CAD build for the part. Positions are in the model's coordinates, mm. A direction names the side the tool comes from. Coordinates: 2 decimals unless noted, no trailing zeros. Order: outer loops, then holes, each group sorted by start corner. A loop starts at its lowest first (then second) coordinate and runs counter-clockwise, first axis right, second up. Notation, with made-up numbers: (69, 68) - (81, 68) arc R30 ccw to (81, 102) - close; hole circle Ø4 at (23, 30.25). An arc over 180 degrees is marked (long way). Use one line per item in the form item = value.
```python
from build123d import *

# Parameters (mm, degrees)
SKETCH030_R             = 14.5
PAD018_DEPTH            = 47
SKETCH031_R             = 1.5875
PAD019_DEPTH            = 15
POCKET012_DEPTH         = 5
SKETCH033_R             = 5.5
PAD020_DEPTH            = 11
SKETCH034_R             = 33.5
PAD021_DEPTH            = 26
SKETCH035_R             = 1.5
POCKET013_DEPTH         = 7.5
SKETCH036_R             = 23
SKETCH036_R_2           = 5.5
POCKET014_DEPTH         = 11
BODY010_PLACEMENT_ANGLE = 180


with BuildPart() as part:
    # Sketch030 → Pad018 (new body)
    with BuildSketch(Plane.XZ):
        Circle(SKETCH030_R)
    extrude(amount=PAD018_DEPTH)

    # Sketch031 → Pad019 (join)
    with BuildSketch(Plane.XZ):
        Circle(SKETCH031_R)
    extrude(amount=-PAD019_DEPTH)

    # Sketch032 → Pocket012 (cut, symmetric)
    with BuildSketch(Plane.YZ):
        Polygon((3, 1.214123), (15, 1.214123), (15, 1.59), (2.863192, 1.59), align=None)
    extrude(amount=POCKET012_DEPTH, both=True, mode=Mode.SUBTRACT)

    # Sketch033 (on Face5 of Pocket012) → Pad020 (join)
    with BuildSketch(Plane(origin=(0, 15, 0), x_dir=(1, 0, 0), z_dir=(0, 1, 0))):
        Circle(SKETCH033_R)
    extrude(amount=-PAD020_DEPTH)

    # Sketch034 (on DatumPlane) → Pad021 (join)
    with BuildSketch(Plane.XZ.offset(-8)):
        Circle(SKETCH034_R)
    extrude(amount=-PAD021_DEPTH)

    # Sketch035 → Pocket013 (cut)
    with BuildSketch(Plane.XZ):
        with Locations((0, -9.5)):
            Circle(SKETCH035_R)
        with Locations((8, 0)):
            Circle(SKETCH035_R)
        with Locations((0, 9.5)):
            Circle(SKETCH035_R)
        with Locations((-8, 0)):
            Circle(SKETCH035_R)
    extrude(amount=POCKET013_DEPTH, mode=Mode.SUBTRACT)

    # Sketch036 (on DatumPlane) → Pocket014 (cut)
    with BuildSketch(Plane.XZ.offset(-8)):
        Circle(SKETCH036_R)
        Circle(SKETCH036_R_2, mode=Mode.SUBTRACT)
    extrude(amount=-POCKET014_DEPTH, mode=Mode.SUBTRACT)


with BuildPart() as part_1:
    # Body010 placement: moved
    add(part.part.moved(Location((-1, -113, 22.5))).rotate(Axis((-1, -113, 22.5), (0, 0, 1)), BODY010_PLACEMENT_ANGLE))


solid = part_1.part
```
Item 1: Cut at C-C, the plane z = 32. Write the cut outline in (x, y), plus the area to 3 significant figures.
Derived:
outline = (-33.12, -147) - (31.12, -147) - (31.12, -121) - (19.95, -121) - (19.95, -132) - (-21.95, -132) - (-21.95, -121) - (-33.12, -121) - close; (-11.95, -113) - (-2.5, -113) - (-2.5, -105.5) - (0.5, -105.5) - (0.5, -113) - (9.95, -113) - (9.95, -66) - (-11.95, -66) - close
area = 2,220 mm²
Item 2: Drop flat-ended pins along their axis: pin 1 (12 mm diameter, centred on x = -22.5, z = 7.5, fed in from +Y); pin 2 (12 mm diameter, centred on x = -13.5, y = -103, fed in from +Z); pin 3 (3 mm diameter, centred on y = -121.5, z = 9, fed in from +X). Give the stop position or say it passes through.
Derived:
pin_1 = -121
pin_2 = 35.46
pin_3 = 30.28
Item 3: Cut at D-D, the plane z = 22.5. Write the cut outline in (x, y).
Derived:
outline = (-34.5, -147) - (32.5, -147) - (32.5, -121) - (22, -121) - (22, -132) - (4.5, -132) - (4.5, -117) - (0.59, -117) - (0.59, -113) - (5.5, -113) - (5.5, -105.5) - (8.5, -105.5) - (8.5, -113) - (13.5, -113) - (13.5, -66) - (-15.5, -66) - (-15.5, -113) - (-10.5, -113) - (-10.5, -105.5) - (-7.5, -105.5) - (-7.5, -113) - (-2.59, -113) - (-2.59, -117) - (-6.5, -117) - (-6.5, -132) - (-24, -132) - (-24, -121) - (-34.5, -121) - close
Item 4: Cut at B-B, the plane x = -5. Write the cut outline in (y, z).
Derived:
outline = (-147, -10.76) - (-121, -10.76) - (-121, -0.15) - (-132, -0.15) - (-132, 18.73) - (-117, 18.73) - (-117, 26.27) - (-132, 26.27) - (-132, 45.15) - (-121, 45.15) - (-121, 55.76) - (-147, 55.76) - close; (-113, 8.56) - (-66, 8.56) - (-66, 36.44) - (-113, 36.44) - close
Item 5: Two-plate mould, pull along X, no slides. Class faces 4 (the face through (1.994, -126.423, 45.304)), 5 (the face through (-32.953, -133.818, 32.562)), 6 (the face through (-2, -117, 24)): +X half, -X half, draft (parallel to the pull), parting line (faces both ways), or undercut.
Derived:
face_4 = undercut
face_5 = parting line
face_6 = draft
Item 6: Cut at A-A, the plane y = -127.5. Write the cut outline in (x, z).
Derived:
outline = circle Ø67 at (-1, 22.5); circle Ø11 at (-1, 22.5); hole circle Ø46 at (-1, 22.5)
Item 7: Drill centre lines: line 1 (Z direction, x = -1, y = -111.25); line 2 (Z direction, x = -1, y = -123); line 3 (Y direction, x = -5, z = 21). Where is each one in solid material? Low to high. Write a range as [from, to].
Derived:
line_1 = [8, 11.5], [14.5, 30.5], [33.5, 37]
line_2 = [-11, -0.5], [17, 28], [45.5, 56]
line_3 = [-147, -117], [-113, -66]
Item 8: 3-axis set-ups, long thin cutter, end or side, ignore diameter. For faces 1 (the face through (-1, -147, 23)), 2 (the face through (-0.284, -124.395, 27.953)), 3 (the face through (0.888, -89.829, 36.877)): which of +Z, -Z, +X, -X, +Y, -Y reach the whole face in a straight line?
Derived:
face_1 = +Z, -Z, +X, -X, -Y
face_2 = none
face_3 = +Y
